```python
from build123d import *

# Parameters (mm, degrees)
EXTRUDE_1_DEPTH = 2


with BuildPart() as part:
    # 草图1 → 凸台-拉伸1 (new body)
    with BuildSketch(Plane.XY):
        Polygon((26.233844386, -52.574512395), (29.233844386, -52.574512395), (29.233844386, -47.574512395), (26.233844386, -47.574512395), (26.233844386, -31.938300989), (44.233844386, 224.125487605), (44.233844386, 233.475487605), (47.233844386, 233.475487605), (47.233844386, 238.475487605), (44.233844386, 238.475487605), (44.233844386, 240.475487605), (41.733844386, 240.475487605), (41.733844386, 238.975487605), (39.133844386, 238.975487605), (39.133844386, 240.475487605), (36.133844386, 240.475487605), (36.133844386, 243.475487605), (39.133844386, 243.475487605), (39.133844386, 244.975487605), (41.733844386, 244.975487605), (41.733844386, 243.475487605), (44.233844386, 243.475487605), (44.233844386, 248.475487605), (44.233844386, 257.475487605), (47.233844386, 257.475487605), (47.233844386, 262.475487605), (44.233844386, 262.475487605), (-48.766155614, 262.475487605), (-51.766155614, 262.475487605), (-51.766155614, 257.475487605), (-48.766155614, 257.475487605), (-48.766155614, 248.475487605), (-48.766155614, 243.475487605), (-46.266155614, 243.475487605), (-46.266155614, 244.975487605), (-43.666155614, 244.975487605), (-43.666155614, 243.475487605), (-40.666155614, 243.475487605), (-40.666155614, 240.475487605), (-43.666155614, 240.475487605), (-43.666155614, 238.975487605), (-46.266155614, 238.975487605), (-46.266155614, 240.475487605), (-48.766155614, 240.475487605), (-48.766155614, 238.475487605), (-51.766155614, 238.475487605), (-51.766155614, 233.475487605), (-48.766155614, 233.475487605), (-48.766155614, 224.125487605), (-30.766155614, -31.938300989), (-30.766155614, -47.574512395), (-33.766155614, -47.574512395), (-33.766155614, -52.574512395), (-30.766155614, -52.574512395), (-30.766155614, -54.574512395), (-28.266155614, -54.574512395), (-28.266155614, -53.074512395), (-25.666155614, -53.074512395), (-25.666155614, -54.574512395), (-22.666155614, -54.574512395), (-22.666155614, -57.574512395), (-25.666155614, -57.574512395), (-25.666155614, -59.074512395), (-28.266155614, -59.074512395), (-28.266155614, -57.574512395), (-30.766155614, -57.574512395), (-30.766155614, -62.574512395), (-33.766155614, -62.574512395), (-33.766155614, -67.574512395), (-30.766155614, -67.574512395), (26.233844386, -67.574512395), (29.233844386, -67.574512395), (29.233844386, -62.574512395), (26.233844386, -62.574512395), (26.233844386, -57.574512395), (23.733844386, -57.574512395), (23.733844386, -59.074512395), (21.133844386, -59.074512395), (21.133844386, -57.574512395), (18.133844386, -57.574512395), (18.133844386, -54.574512395), (21.133844386, -54.574512395), (21.133844386, -53.074512395), (23.733844386, -53.074512395), (23.733844386, -54.574512395), (26.233844386, -54.574512395), align=None)
        with BuildLine():
            Line((-17.266155614, -1.672218314), (-17.266155614, 65.795616335))
            ThreePointArc((-17.266155614, 65.795616335), (-2.266155614, 80.795616335), (12.733844386, 65.795616335))
            Line((12.733844386, 65.795616335), (12.733844386, -1.672218314))
            ThreePointArc((12.733844386, -1.672218314), (-2.266155614, -16.672218314), (-17.266155614, -1.672218314))
        make_face(mode=Mode.SUBTRACT)
        with BuildLine():
            Line((-22.266155614, 216.327781686), (-22.266155614, 126.327781686))
            ThreePointArc((-22.266155614, 126.327781686), (-2.266155614, 106.327781686), (17.733844386, 126.327781686))
            Line((17.733844386, 126.327781686), (17.733844386, 216.327781686))
            ThreePointArc((17.733844386, 216.327781686), (-2.266155614, 236.327781686), (-22.266155614, 216.327781686))
        make_face(mode=Mode.SUBTRACT)
    extrude(amount=EXTRUDE_1_DEPTH)


solid = part.part
```
Verification items for the finished model (mm, model axes). A direction names the side the tool comes from. Coordinates: 2 decimals unless noted, no trailing zeros. Loops run counter-clockwise (first coordinate to the right, second up) from the corner with the lowest first, then second, coordinate; pieces in that order, holes last. Notation, with made-up numbers: (-18.5, 68.25) - (30.5, 68.25) arc R16 ccw to (30.5, 81.25) - close; hole circle Ø6 at (51.5, 68.25). An arc over 180 degrees is marked (long way). Return JSON: item names as keys, results as strings.
1. Thickness scan on L1, parallel to X at y = 239.5, z = 1.6; L2, parallel to X at y = -53.5, z = 0.7; L3, parallel to Y at x = -10, z = 0.8. Record the ranges inside material, lowest first.
Established:
{"L1": "x = -48.77 to -46.27, -43.67 to 39.13, 41.73 to 44.23", "L2": "x = -30.77 to -28.27, -25.67 to 21.13, 23.73 to 26.23", "L3": "y = -67.57 to -14.52, 78.65 to 107.88, 234.77 to 262.48"}
2. Go/stop test with flat-tipped pins: pin 1 (1.2 mm diameter, centred on y = -58, z = 1.5, fed in from -X); pin 2 (1 mm diameter, centred on y = 148, z = 2, fed in from +X); pin 3 (0.6 mm diameter, centred on y = 242.5, z = 1.5, fed in from +X). Record where each tip stops, or that it passes through.
Established:
{"pin 1": "stops at x = -30.77", "pin 2": "stops at x = 38.92", "pin 3": "stops at x = 36.13"}
3. Mould release check, pull along Y, two halves, no side actions. Record for faces 1 (the cylindrical face through (-2.706, 106.333, 0.986)), 2 (the flat face through (19, 136, 2)): +Y half, -Y half, draft (parallel to the pull), parting line (faces both ways), or undercut.
Established:
{"face 1": "undercut", "face 2": "draft"}
4. Tool access check on faces 3 (the flat face through (19, 136, 0)), 4 (the flat face through (35.108, 94.301, 0.986)), 5 (the cylindrical face through (-1.94, -16.67, 0.99)). Record the directions out of +Z, -Z, +X, -X, +Y, -Y that give a thin tool (end or side, any length) a straight path to the whole face; none if there is none.
Established:
{"face 3": "-Z, +X, -X, +Y, -Y", "face 4": "+Z, -Z, +X", "face 5": "+Z, -Z"}
5. Section check D-D, the plane y = 185. Record the boundary of the cut face in (x, z), then the cut area to 3 significant figures.
Established:
{"outline": "(-46.02, 0) - (-22.27, 0) - (-22.27, 2) - (-46.02, 2) - close; (17.73, 0) - (41.48, 0) - (41.48, 2) - (17.73, 2) - close", "area": "95.0 mm2"}
6. Section check C-C, the plane z = 0.55. Count the separate pieces of the cut face and the enclosed holes in it, then the cut area to 3 significant figures.
Established:
{"separate pieces": "1", "enclosed holes": "2", "area": "17,200 mm2"}
7. Section check B-B, the plane y = 27. Record the boundary of the cut face in (x, z), then the cut area to 3 significant figures.
Established:
{"outline": "(-34.91, 0) - (-17.27, 0) - (-17.27, 2) - (-34.91, 2) - close; (12.73, 0) - (30.38, 0) - (30.38, 2) - (12.73, 2) - close", "area": "70.6 mm2"}
8. Section check A-A, the plane x = -13. Record the boundary of the cut face in (y, z).
Established:
{"outline": "(-67.57, 0) - (-12.15, 0) - (-12.15, 2) - (-67.57, 2) - close; (76.27, 0) - (109.45, 0) - (109.45, 2) - (76.27, 2) - close; (233.2, 0) - (262.48, 0) - (262.48, 2) - (233.2, 2) - close"}
